Design review of the part built by this model. Coordinates are the model's own, in mm. A direction names the side the tool comes from. Round coordinates to 2 decimals unless told otherwise and drop trailing zeros. Order: outer loops, then holes, each group sorted by start corner. A loop starts at its lowest first (then second) coordinate and runs counter-clockwise, first axis right, second up. Notation, with made-up numbers: M 0.25,-27.5 L 58.25,-27.5 A32 ccw 58.25,7.5 Z; hole C -20,44 d2. An arc over 180 degrees is marked long. Use a Markdown table: item, result. Add a question column.
(1) The part is to be moulded in two halves that separate along Y. For faces 4 (the face through (5, 11, 2.032)), 5 (the face through (6, 14.605, -4)), 6 (the face through (5.461, 11, -4)), say which applies: released by +Y, released by -Y, zero draft, split by the parting line, or undercut.
(2) Take a section at C-C (y = 2.5). Write out the cut boundary in (x, z) (3 decimals).
(3) Machinability: for faces 1 (the face through (0, 7, -4)), 2 (the face through (6, 2, 0.127)), 3 (the face through (10.922, 6, -4)), which of the approach directions +Z, -Z, +X, -X, +Y, -Y give a long, thin tool a straight path to every point of the face, cutting with its end or side? Answer none if there is none.
(4) For pin 1 (0.6 mm diameter, centred on x = 6, z = -4.5, fed in from -Y); pin 2 (5 mm diameter, centred on x = 8, y = 6.5, fed in from +Z); pin 3 (2 mm diameter, centred on x = 9, y = 2, fed in from +Z), all flat-tipped, find the tip position at first contact; note any pin that passes through.
(5) Take a section at B-B (x = 7.5). Write out the cut boundary in (y, z) (3 decimals).
(6) To check wall thickness, follow probe 1 along Y at (x, z) = (2, -8.5) (3 decimals); probe 2 along X at (y, z) = (8.75, -6.5) (3 decimals); probe 3 along Y at (x, z) = (6.5, -8.25) (3 decimals). State the ranges of each line that lie inside material, in increasing order. Write a range as from..to.
(7) Take a section at A-A (z = -4). Write out the cut boundary in (x, y) (3 decimals), then the cut area to 3 significant figures.
(8) Take a section at D-D (x = 6.25). Write out the cut boundary in (y, z) (3 decimals).
```python
from build123d import *

# Parameters (mm, degrees)
EXTRUDE1_DEPTH = 2.032
SKETCH2_W      = 9.8552
SKETCH2_H      = 2.54
EXTRUDE3_DEPTH = 11.303
SKETCH3_W      = 9.8552
SKETCH3_H      = 2.54
EXTRUDE4_DEPTH = 1.905
SKETCH4_W      = 12.065
SKETCH4_H      = 14.605
EXTRUDE5_DEPTH = 1.905


with BuildPart() as part:
    # Sketch1 → Extrude1 (new body)
    with BuildSketch(Plane.XY):
        Polygon((0, 0), (0, 14.605), (12.065, 14.605), (12.065, 0), (10.922, 0), (10.922, 11.938), (9.779, 11.938), (9.779, 13.462), (6.604, 13.462), (6.604, 11.938), (5.461, 11.938), (5.461, 10.16), (1.0668, 10.16), (1.0668, 0), align=None)
    extrude(amount=EXTRUDE1_DEPTH)

    # Sketch2 → Extrude3 (add)
    with BuildSketch(Plane.XY.offset(2.032)):
        Polygon((0, 14.605), (0, 0), (1.0668, 0), (1.0668, 10.16), (5.461, 10.16), (5.461, 11.938), (6.604, 11.938), (6.604, 13.462), (9.779, 13.462), (9.779, 11.938), (10.922, 11.938), (10.922, 0), (12.065, 0), (12.065, 14.605), align=None)
        with Locations((5.9944, 2.0701)):
            Rectangle(SKETCH2_W, SKETCH2_H)
    extrude(amount=-EXTRUDE3_DEPTH)

    # Sketch3 → Extrude4 (cut)
    with BuildSketch(Plane.XY.offset(2.032)):
        with Locations((5.9944, 2.0701)):
            Rectangle(SKETCH3_W, SKETCH3_H)
    extrude(amount=-EXTRUDE4_DEPTH, mode=Mode.SUBTRACT)

    # Sketch4 → Extrude5 (add)
    with BuildSketch(Plane(origin=(0, 0, -9.271), x_dir=(-1, 0, 0), z_dir=(0, 0, -1))):
        with Locations((-6.0325, 7.3025)):
            Rectangle(SKETCH4_W, SKETCH4_H)
    extrude(amount=EXTRUDE5_DEPTH)


solid = part.part
```
Verdict:
| question | item | result |
|---|---|---|
| 1 | face 4 | zero draft |
| 1 | face 5 | released by +Y |
| 1 | face 6 | undercut |
| 2 | outline | M 0,-11.176 L 12.065,-11.176 L 12.065,2.032 L 10.922,2.032 L 10.922,0.127 L 1.067,0.127 L 1.067,2.032 L 0,2.032 Z |
| 3 | face 1 | +Z, -Z, -X, +Y, -Y |
| 3 | face 2 | +Z, -Y |
| 3 | face 3 | +Z |
| 4 | pin 1 | stops at y = 0.8 |
| 4 | pin 2 | stops at z = -9.27 |
| 4 | pin 3 | stops at z = 0.13 |
| 5 | outline | M 0,-11.176 L 14.605,-11.176 L 14.605,2.032 L 13.462,2.032 L 13.462,-9.271 L 3.34,-9.271 L 3.34,0.127 L 0.8,0.127 L 0.8,-9.271 L 0,-9.271 Z |
| 6 | probe 1 | y = 0.8..3.34, 10.16..14.605 |
| 6 | probe 2 | x = 0..1.067, 10.922..12.065 |
| 6 | probe 3 | y = 0.8..3.34, 11.938..14.605 |
| 7 | outline | M 0,0 L 1.067,0 L 1.067,0.8 L 10.922,0.8 L 10.922,0 L 12.065,0 L 12.065,14.605 L 0,14.605 Z; hole M 1.067,3.34 L 10.922,3.34 L 10.922,11.938 L 9.779,11.938 L 9.779,13.462 L 6.604,13.462 L 6.604,11.938 L 5.461,11.938 L 5.461,10.16 L 1.067,10.16 Z |
| 7 | area | 86.6 mm^2 |
| 8 | outline | M 0,-11.176 L 14.605,-11.176 L 14.605,2.032 L 11.938,2.032 L 11.938,-9.271 L 3.34,-9.271 L 3.34,0.127 L 0.8,0.127 L 0.8,-9.271 L 0,-9.271 Z |
